Could you check a few things on this model? Use its own coordinates, in mm. A direction names the side the tool comes from. Round coordinates to 2 decimals unless told otherwise and drop trailing zeros. Write each loop counter-clockwise with the first axis right and the second up, starting at its lowest first coordinate (ties: lowest second). Pieces come first, ordered by that corner, then holes. Notation, with made-up numbers: (34, 43) - (74, 43) arc R14 ccw to (74, 63) - close; hole circle Ø3 at (14.25, -27). An arc over 180 degrees is marked (long way). Put each result on its own line as item: value.
from build123d import *

# Parameters (mm, degrees)
SKETCH_187_R    = 2.75
SKETCH_187_R_2  = 1.35
EXTRUDE_1_DEPTH = 2


with BuildPart() as part:
    # Sketch 187 → 凸台-拉伸1 (new body)
    with BuildSketch(Plane.XY):
        with BuildLine():
            Line((-24.447800114, 142.867788384), (-29.015821613, 138.834288737))
            ThreePointArc((-29.015821613, 138.834288737), (-30.556091587, 137.905760103), (-32.325263946, 137.582300402))
            Line((-32.325263946, 137.582300402), (-39.033457742, 137.582300402))
            ThreePointArc((-39.033457742, 137.582300402), (-40.802630101, 137.2588407), (-42.342900075, 136.330312067))
            Line((-42.342900075, 136.330312067), (-44.480254451, 134.443057788))
            ThreePointArc((-44.480254451, 134.443057788), (-45.728619247, 132.750865708), (-46.170812117, 130.695046123))
            Line((-46.170812117, 130.695046123), (-46.170812117, 100.244585214))
            ThreePointArc((-46.170812117, 100.244585214), (-45.11839985, 97.487233211), (-42.496431366, 96.132300402))
            Line((-42.496431366, 96.132300402), (-34.05, 95.17927075))
            Line((-34.05, 95.17927075), (-29.442356392, 90.712497735))
            Line((-29.442356392, 90.712497735), (-29.442356392, 87.789843939))
            Line((-29.442356392, 87.789843939), (-19.688242157, 78.763336754))
            Line((-19.688242157, 78.763336754), (-14.532154357, 78.763336754))
            Line((-14.532154357, 78.763336754), (-9.532154357, 83.763336754))
            Line((-9.532154357, 83.763336754), (9.532154357, 83.763336754))
            Line((9.532154357, 83.763336754), (14.532154357, 78.763336754))
            Line((14.532154357, 78.763336754), (19.688242157, 78.763336754))
            Line((19.688242157, 78.763336754), (29.442356392, 87.789843939))
            Line((29.442356392, 87.789843939), (29.442356392, 90.712497735))
            Line((29.442356392, 90.712497735), (34.05, 95.17927075))
            Line((34.05, 95.17927075), (42.496431366, 96.132300402))
            ThreePointArc((42.496431366, 96.132300402), (45.11839985, 97.487233211), (46.170812117, 100.244585214))
            Line((46.170812117, 100.244585214), (46.170812117, 130.695046123))
            ThreePointArc((46.170812117, 130.695046123), (45.728619247, 132.750865708), (44.480254451, 134.443057788))
            Line((44.480254451, 134.443057788), (42.342900075, 136.330312067))
            ThreePointArc((42.342900075, 136.330312067), (40.802630101, 137.2588407), (39.033457742, 137.582300402))
            Line((39.033457742, 137.582300402), (32.472417217, 137.582300402))
            ThreePointArc((32.472417217, 137.582300402), (30.584617738, 137.952374579), (28.976268595, 139.007815151))
            Line((28.976268595, 139.007815151), (25.245537252, 142.656785653))
            ThreePointArc((25.245537252, 142.656785653), (23.637188108, 143.712226225), (21.74938863, 144.082300402))
            Line((21.74938863, 144.082300402), (15.032154357, 144.082300402))
            Line((15.032154357, 144.082300402), (9.532154357, 138.582300402))
            Line((9.532154357, 138.582300402), (-9.532154357, 138.582300402))
            Line((-9.532154357, 138.582300402), (-15.032154357, 144.082300402))
            Line((-15.032154357, 144.082300402), (-21.74938863, 144.082300402))
            ThreePointArc((-21.74938863, 144.082300402), (-23.190499918, 143.679240794), (-24.447800114, 142.867788384))
        make_face()
        with Locations((39.335406059, 129.082300402)):
            Circle(SKETCH_187_R, mode=Mode.SUBTRACT)
        with Locations((39.335406059, 104.082300402)):
            Circle(SKETCH_187_R, mode=Mode.SUBTRACT)
        with Locations((17.23796389, 84.763336754)):
            Circle(SKETCH_187_R, mode=Mode.SUBTRACT)
        with Locations(Location((-17.23796389, 84.763336754, 0), (0, 0, 180))):
            Circle(SKETCH_187_R, mode=Mode.SUBTRACT)
        with Locations(Location((-39.335406059, 104.082300402, 0), (0, 0, 180))):
            Circle(SKETCH_187_R, mode=Mode.SUBTRACT)
        with Locations(Location((-39.335406059, 129.082300402, 0), (0, 0, 180))):
            Circle(SKETCH_187_R, mode=Mode.SUBTRACT)
        with Locations(Location((24.85, 129.082300402, 0), (0, 0, 180))):
            Circle(SKETCH_187_R, mode=Mode.SUBTRACT)
        with Locations((-24.85, 129.082300402)):
            Circle(SKETCH_187_R, mode=Mode.SUBTRACT)
        with Locations(Location((-24.85, 104.082300402, 0), (0, 0, 180))):
            Circle(SKETCH_187_R, mode=Mode.SUBTRACT)
        with Locations((24.85, 104.082300402)):
            Circle(SKETCH_187_R, mode=Mode.SUBTRACT)
        with Locations((12.5, 131.582300402)):
            Circle(SKETCH_187_R_2, mode=Mode.SUBTRACT)
        with Locations(Location((-12.5, 131.582300402, 0), (0, 0, 180))):
            Circle(SKETCH_187_R_2, mode=Mode.SUBTRACT)
        with Locations((-12.5, 101.582300402)):
            Circle(SKETCH_187_R_2, mode=Mode.SUBTRACT)
        with Locations(Location((12.5, 101.582300402, 0), (0, 0, 180))):
            Circle(SKETCH_187_R_2, mode=Mode.SUBTRACT)
        Polygon((7.105388598, 96.132300402), (-7.105388598, 96.132300402), (-9.761471208, 92.339021317), (-9.761471208, 90.339021317), (9.761471208, 90.339021317), (9.761471208, 92.339021317), align=None, mode=Mode.SUBTRACT)
        with BuildLine():
            Line((-35.6, 116.582300402), (-35.6, 112.082300402))
            ThreePointArc((-35.6, 112.082300402), (-34.05, 110.532300402), (-32.5, 112.082300402))
            Line((-32.5, 112.082300402), (-32.5, 116.582300402))
            ThreePointArc((-32.5, 116.582300402), (-34.05, 118.132300402), (-35.6, 116.582300402))
        make_face(mode=Mode.SUBTRACT)
        with BuildLine():
            Line((35.6, 116.582300402), (35.6, 112.082300402))
            ThreePointArc((35.6, 112.082300402), (34.05, 110.532300402), (32.5, 112.082300402))
            Line((32.5, 112.082300402), (32.5, 116.582300402))
            ThreePointArc((32.5, 116.582300402), (34.05, 118.132300402), (35.6, 116.582300402))
        make_face(mode=Mode.SUBTRACT)
        with BuildLine():
            Line((6.033287824, 125.625579487), (-5.574654121, 125.625579487))
            ThreePointArc((-5.574654121, 125.625579487), (-6.729025654, 125.34310657), (-7.622534231, 124.559520578))
            Line((-7.622534231, 124.559520578), (-9.532154357, 121.832300402))
            Line((-9.532154357, 121.832300402), (-9.532154357, 119.832300402))
            Line((-9.532154357, 119.832300402), (9.99078806, 119.832300402))
            Line((9.99078806, 119.832300402), (9.99078806, 121.832300402))
            Line((9.99078806, 121.832300402), (8.081167934, 124.559520578))
            ThreePointArc((8.081167934, 124.559520578), (7.187659357, 125.34310657), (6.033287824, 125.625579487))
        make_face(mode=Mode.SUBTRACT)
    extrude(amount=EXTRUDE_1_DEPTH)


solid = part.part
(1) Imagine slicing it at B-B, the plane y = 94. List the corners of the cut face in (x, z) for me, then the cut area to 3 significant figures.
Values found:
outline: (-32.83, 0) - (-8.6, 0) - (-8.6, 2) - (-32.83, 2) - close; (8.6, 0) - (32.83, 0) - (32.83, 2) - (8.6, 2) - close
area: 96.9 mm^2
(2) I'm going to push flat-ended pins straight in: pin 1 (1 mm diameter, centred on y = 90, z = 0.5, fed in from -X); pin 2 (1 mm diameter, centred on x = -35, z = 0.5, fed in from +Y); pin 3 (4.5 mm diameter, centred on x = 39.34, y = 129.08, fed in from -Z). Where does each tip first touch, or does it pass through?
Values found:
pin 1: stops at x = -29.44
pin 2: stops at y = 137.58
pin 3: passes through
(3) Please list where these lines run through material, in increasing order: probe 1 along Y at (x, z) = (0, 0.5); probe 2 along X at (y, z) = (129, 1.2); probe 3 along Y at (x, z) = (38, 1.8). Write a range as from..to.
Values found:
probe 1: y = 83.76..90.34, 96.13..119.83, 125.63..138.58
probe 2: x = -46.17..-42.08, -36.59..-27.6, -22.1..22.1, 27.6..36.59, 42.08..46.17
probe 3: y = 95.62..101.68, 106.49..126.68, 131.49..137.58
(4) If we mould it in two halves opening along X, with no side actions, what happens to faces 1 (the face through (43.43, 135.37, 0.99)), 2 (the face through (-25.21, 131.81, 0.99)), 3 (the face through (-23.17, 143.69, 0.99))? For each: pulls with the +X half, pulls with the -X half, needs draft (parallel to the pull), parting line crosses it, or undercut.
Values found:
face 1: pulls with the +X half
face 2: undercut
face 3: pulls with the -X half
(5) Imagine slicing it at A-A, the plane x = 4. List the corners of the cut face in (y, z) for me.
Values found:
outline: (83.76, 0) - (90.34, 0) - (90.34, 2) - (83.76, 2) - close; (96.13, 0) - (119.83, 0) - (119.83, 2) - (96.13, 2) - close; (125.63, 0) - (138.58, 0) - (138.58, 2) - (125.63, 2) - close
(6) Imagine slicing it at C-C, the plane z = 1.65. Give the number of separate pieces and of enclosed holes in the cut face, then the cut area to 3 significant figures.
Values found:
separate pieces: 1
enclosed holes: 18
area: 4,350 mm^2
(7) For faces 4 (the face through (-30.532, 137.915, 0.986)), 5 (the face through (-6.714, 125.351, 0.986)), 6 (the face through (36, 137.582, 1)), which set-ups out of +Z, -Z, +X, -X, +Y, -Y let a thin tool reach every point of the face, with its end or its side?
Values found:
face 4: +Z, -Z, -X, +Y
face 5: +Z, -Z
face 6: +Z, -Z, +X, +Y
(8) Imagine slicing it at D-D, the plane x = -12.5. List the corners of the cut face in (y, z) for me, then the cut area to 3 significant figures.
Values found:
outline: (80.8, 0) - (100.23, 0) - (100.23, 2) - (80.8, 2) - close; (102.93, 0) - (130.23, 0) - (130.23, 2) - (102.93, 2) - close; (132.93, 0) - (141.55, 0) - (141.55, 2) - (132.93, 2) - close
area: 111 mm^2
